```python
from build123d import *

# Parameters (mm, degrees)
F0_R     = 6.1702881354
F1_DEPTH = 10.24551
F2_DEPTH = 19.44125
F3_DEPTH = 12.29025


# Not quite as in the source:
# - the program builds the solid bodies; features that only make, move or delete a surface that nothing else refers to are left out


with BuildPart() as f1:
    # F0 (on Front) → F1 (new body)
    with BuildSketch(Plane.XZ):
        with BuildLine():
            ThreePointArc((7.9096967883, -9.6482263274), (5.7944386046, 0), (7.9096967883, 9.6482263274))
            add(Edge.make_bspline(
                [(7.9096967883, 9.6482263274), (7.1691805882, 8.7133229845), (4.8849042306, 7.0496072248), (1.7047020698, 7.2518519174), (0, 7.3653594591)],
                knots=[0.305255717, 0.305255717, 0.305255717, 0.305255717, 0.6293542053, 1, 1, 1, 1], degree=3))
            Line((0, 7.3653594591), (-27.2417403758, 7.3653594591))
            ThreePointArc((-27.2417403758, 7.3653594591), (-35.1115765516, -0.5044767167), (-27.2417403758, -8.3743128926))
            Line((-27.2417403758, -8.3743128926), (0, -8.3743128926))
            add(Edge.make_bspline(
                [(7.9096967883, -9.6482263274), (7.1553998901, -8.8616436412), (4.7881379326, -7.7629787373), (1.6803783566, -8.1685536627), (0, -8.3743128926)],
                knots=[0.3094407552, 0.3094407552, 0.3094407552, 0.3094407552, 0.6242726729, 1, 1, 1, 1], degree=3))
        make_face()
        with Locations((-27.2417403758, -0.5044767167)):
            Circle(F0_R, mode=Mode.SUBTRACT)
    extrude(amount=F1_DEPTH)

    # F0 (on Front) → F2 (join)
    with BuildSketch(Plane.XZ):
        with BuildLine():
            Line((29.1485549066, 14.2256355643), (47.0073711523, 14.2256355643))
            ThreePointArc((47.0073711523, 14.2256355643), (40.9442597431, 19.6396071394), (33.3793842605, 22.6136728933))
            Line((33.3793842605, 22.6136728933), (33.3793842605, 18.8674259181))
            Line((33.3793842605, 18.8674259181), (25.0220429152, 18.8674259181))
            Line((25.0220429152, 18.8674259181), (25.0220429152, 22.7406880158))
            ThreePointArc((25.0220429152, 22.7406880158), (16.1840833933, 19.2680953065), (9.494543791, 12.5287712643))
            add(Edge.make_bspline(
                [(9.494543791, 12.5287712643), (9.0162268309, 11.5501776901), (8.6071600956, 10.5287752978), (7.9096967883, 9.6482263274)],
                knots=[0, 0, 0, 0, 0.305255717, 0.305255717, 0.305255717, 0.305255717], degree=3))
            ThreePointArc((7.9096967883, 9.6482263274), (5.7944386046, 0), (7.9096967883, -9.6482263274))
            add(Edge.make_bspline(
                [(9.494543791, -12.5287712643), (9.0785331078, -11.4704442228), (8.6510771527, -10.4213396199), (7.9096967883, -9.6482263274)],
                knots=[0, 0, 0, 0, 0.3094407552, 0.3094407552, 0.3094407552, 0.3094407552], degree=3))
            ThreePointArc((9.494543791, -12.5287712643), (16.441223865, -19.434771268), (25.6276700044, -22.8345370586))
            Line((25.6276700044, -22.8345370586), (25.6276700044, -18.9136881421))
            Line((25.6276700044, -18.9136881421), (33.3589574797, -18.8714867898))
            Line((33.3589574797, -18.8714867898), (33.3793842605, -22.6136728933))
            ThreePointArc((33.3793842605, -22.6136728933), (40.9439316742, -19.6398090623), (47.0068958817, -14.2262419686))
            Line((47.0068958817, -14.2262419686), (29.2007135878, -14.2262419686))
            Line((29.2007135878, -14.2262419686), (28.8560651243, -3.7142947274))
            Line((28.8560651243, -3.7142947274), (13.5199762881, -3.7142947274))
            Line((13.5199762881, -3.7142947274), (13.5199762881, 4.6701654948))
            Line((13.5199762881, 4.6701654948), (29.2007135878, 4.6701654948))
            Line((29.2007135878, 4.6701654948), (29.1485549066, 14.2256355643))
        make_face()
    extrude(amount=F2_DEPTH)

    # F0 (on Front) → F3 (join)
    with BuildSketch(Plane.XZ):
        with BuildLine():
            ThreePointArc((47.0068958817, -14.2262419686), (49.9762101479, -9.2616462852), (51.6166150388, -3.7142947274))
            Line((51.6166150388, -3.7142947274), (28.8560651243, -3.7142947274))
            Line((28.8560651243, -3.7142947274), (29.2007135878, -14.2262419686))
            Line((29.2007135878, -14.2262419686), (47.0068958817, -14.2262419686))
        make_face()
        with BuildLine():
            Line((29.2007135878, 4.6701654948), (51.4398684351, 4.6701654948))
            ThreePointArc((51.4398684351, 4.6701654948), (49.7764866132, 9.704358941), (47.0073711523, 14.2256355643))
            Line((47.0073711523, 14.2256355643), (29.1485549066, 14.2256355643))
            Line((29.1485549066, 14.2256355643), (29.2007135878, 4.6701654948))
        make_face()
    extrude(amount=F3_DEPTH)


solid = f1.part
```
Model file for the job. Use its own axes, mm. A direction names the side the tool comes from. Give positions to 0.01 mm unless a question says otherwise; leave off trailing zeros. Loops run counter-clockwise (first coordinate to the right, second up) from the corner with the lowest first, then second, coordinate; pieces in that order, holes last. Notation, with made-up numbers: (89, 59) - (142, 59) arc R34 ccw to (142, 90) - close; hole circle Ø3 at (86.5, 15). An arc over 180 degrees is marked (long way). One line per item, written item: value. Start each with the question number.
1. Pin check, flat tips, straight feed: pin 1 (6 mm diameter, centred on y = -2.5, z = 13.5, fed in from -X); pin 2 (9.5 mm diameter, centred on x = -23.5, z = -2.5, fed in from -Y); pin 3 (1.2 mm diameter, centred on y = -8.5, z = 21.5, fed in from +X); pin 4 (1 mm diameter, centred on x = -21, z = 9.5, fed in from -Y). Stop position of each tip, or through.
2. Which spindle directions (+Z, -Z, +X, -X, +Y, -Y) get a long thin tool onto all of the face, cutting with end or side? Do faces 1 (the flat face through (25.628, -10, -21)), 2 (the flat face through (38, -16, 14.226)), 3 (the flat face through (-13, -5, 7.365)), 4 (the flat face through (-14, -5, -8.374)), 5 (the flat face through (13.52, -10, 0)). Say none if no direction does.
3. Probe L1, parallel to Z at x = 33, y = -9.75; L2, parallel to Y at x = 45.5, z = 10.5; L3, parallel to X at y = -2, z = -0.5. List the from-to ranges inside material, lowest first. Write a range as from..to.
4. Slice it at C-C (x = -24.5). List the corners of the cut face in (y, z).
5. Slice it at A-A (x = 21). List the corners of the cut face in (y, z).
6. Slice it at B-B (z = -5). List the corners of the cut face in (x, y).
7. Pull direction X, two halves, no side cores. Call faces 6 (the flat face through (32, -7, 4.67)), 7 (the flat face through (29, -10, 18.867)), 8 (the cylindrical face through (16.325, -9.585, -19.36)): pulls with the +X half, pulls with the -X half, needs draft (parallel to the pull), parting line crosses it, or undercut.
8. Slice it at D-D (x = 39). List the corners of the cut face in (y, z).
Solution:
1. pin 1: stops at x = 8.48
1. pin 2: stops at y = -10.25
1. pin 3: stops at x = 38.6
1. pin 4: passes through
2. face 1: -Z, +Y, -Y
2. face 2: +X, -Y
2. face 3: +Z, -X, +Y, -Y
2. face 4: -Z, -X, +Y, -Y
2. face 5: +X, +Y, -Y
3. L1: z = -18.87..-3.71, 4.67..18.87
3. L2: y = -12.29..0
3. L3: x = -35.11..-33.41, -21.07..13.52
4. outline: (-10.25, -8.37) - (0, -8.37) - (0, -6.03) - (-10.25, -6.03) - close; (-10.25, 5.02) - (0, 5.02) - (0, 7.37) - (-10.25, 7.37) - close
5. outline: (-19.44, -21.68) - (0, -21.68) - (0, -3.71) - (-19.44, -3.71) - close; (-19.44, 4.67) - (0, 4.67) - (0, 21.68) - (-19.44, 21.68) - close
6. outline: (-33.7, -10.25) - (-31.47, -10.25) - (-31.47, 0) - (-33.7, 0) - close; (-23.02, -10.25) - (6.34, -10.25) - (6.34, -19.44) - (28.9, -19.44) - (28.9, -12.29) - (51.37, -12.29) - (51.37, 0) - (-23.02, 0) - close
7. face 6: needs draft
7. face 7: undercut
7. face 8: pulls with the -X half
8. outline: (-19.44, -20.71) - (0, -20.71) - (0, -3.71) - (-12.29, -3.71) - (-12.29, -14.23) - (-19.44, -14.23) - close; (-19.44, 14.23) - (-12.29, 14.23) - (-12.29, 4.67) - (0, 4.67) - (0, 20.71) - (-19.44, 20.71) - close
